Part model, mm, in its own coordinate system. A direction names the side the tool comes from. Round coordinates to 2 decimals unless told otherwise and drop trailing zeros. Loops run counter-clockwise (first coordinate to the right, second up) from the corner with the lowest first, then second, coordinate; pieces in that order, holes last. Notation, with made-up numbers: M -32.5,68.25 L -18.5,68.25 A17 cw -18.5,77.25 Z; hole C 86,41.25 d6. An arc over 180 degrees is marked long. Put each result on its own line as item: value. Start each with the question number.
1) Slice it at C-C on y = 351. Give the cut face in (x, z), then the cut area to 3 significant figures.
2) Drop flat-ended pins along their axis: pin 1 Ø1.2 at (y, z) = (12.5, -0.5) entering from -X; pin 2 Ø3.5 at (x, y) = (29.5, 930) entering from +Z; pin 3 Ø12 at (x, z) = (7, -27) entering from -Y. Give the stop position or say it passes through.
3) Which spindle directions (+Z, -Z, +X, -X, +Y, -Y) get a long thin tool onto all of the face, cutting with end or side? Do faces 1 (the flat face through (1, 20, -20)), 2 (the flat face through (38.5, 602, -20)), 3 (the flat face through (1, 1200, -20)), 4 (the flat face through (20, 601, 0)), 5 (the flat face through (0, 602, -20)). Say none if no direction does.
4) Pull direction X, two halves, no side cores. Call faces 6 (the flat face through (20, 601, -40)), 7 (the flat face through (40, 602, -20)), 8 (the flat face through (20, 601, -1.5)): +X half, -X half, draft (parallel to the pull), parting line (faces both ways), or undercut.
5) Slice it at B-B on z = -28.5. Give the cut face in (x, y), then the cut area to 3 significant figures.
6) Slice it at A-A on x = 13.5. Give the cut face in (y, z), then the cut area to 3 significant figures.
7) Probe line 1 along Z through (x, y) = (7, 613.5); line 2 along X through (y, z) = (69, -11); line 3 along X through (y, z) = (730, -1.1). List the from-to ranges inside material, lowest first.
```python
from build123d import *

# Parameters (mm, degrees)
SKETCH1_W           = 37
SKETCH1_H           = 37
BOSS_EXTRUDE1_DEPTH = 1220
SKETCH2_W           = 20
SKETCH2_H           = 20
SKETCH2_W_2         = 5
CUT_EXTRUDE1_DEPTH  = 50
SKETCH3_R           = 3
CUT_EXTRUDE2_DEPTH  = 10


with BuildPart() as part:
    # Sketch1 → Boss-Extrude1 (new body)
    with BuildSketch(Plane(origin=(0, 0, 0), x_dir=(1, 0, 0), z_dir=(0, 1, 0))):
        with BuildLine():
            Line((0.5, 0), (39.5, 0))
            ThreePointArc((39.5, 0), (39.853553391, 0.146446609), (40, 0.5))
            Line((40, 0.5), (40, 39.5))
            ThreePointArc((40, 39.5), (39.853553391, 39.853553391), (39.5, 40))
            Line((39.5, 40), (0.5, 40))
            ThreePointArc((0.5, 40), (0.146446609, 39.853553391), (0, 39.5))
            Line((0, 39.5), (0, 0.5))
            ThreePointArc((0, 0.5), (0.146446609, 0.146446609), (0.5, 0))
        make_face()
        with Locations((20, 20)):
            Rectangle(SKETCH1_W, SKETCH1_H, mode=Mode.SUBTRACT)
    extrude(amount=BOSS_EXTRUDE1_DEPTH)

    # Sketch2 → Cut-Extrude1 (cut)
    with BuildSketch(Plane.XY):
        with Locations((10, 1210)):
            Rectangle(SKETCH2_W, SKETCH2_H)
        with Locations((37.5, 1210)):
            Rectangle(SKETCH2_W_2, SKETCH2_H)
        with Locations((10, 10)):
            Rectangle(SKETCH2_W, SKETCH2_H)
        with Locations((37.5, 10)):
            Rectangle(SKETCH2_W_2, SKETCH2_H)
    extrude(amount=-CUT_EXTRUDE1_DEPTH, mode=Mode.SUBTRACT)

    # Sketch3 → Cut-Extrude2 (cut)
    with BuildSketch(Plane.XY):
        with Locations((29.5, 90)):
            Circle(SKETCH3_R)
        with Locations((29.5, 290)):
            Circle(SKETCH3_R)
        with Locations((29.5, 490)):
            Circle(SKETCH3_R)
        with Locations(Location((29.5, 730, 0), (0, 0, 180))):
            Circle(SKETCH3_R)
        with Locations(Location((29.5, 930, 0), (0, 0, 180))):
            Circle(SKETCH3_R)
        with Locations(Location((29.5, 1130, 0), (0, 0, 180))):
            Circle(SKETCH3_R)
    extrude(amount=-CUT_EXTRUDE2_DEPTH, mode=Mode.SUBTRACT)


solid = part.part
```
Recorded:
1. outline: M 0,-39.5 A0.5 ccw 0.5,-40 L 39.5,-40 A0.5 ccw 40,-39.5 L 40,-0.5 A0.5 ccw 39.5,0 L 0.5,0 A0.5 ccw 0,-0.5 Z; hole M 1.5,-38.5 L 38.5,-38.5 L 38.5,-1.5 L 1.5,-1.5 Z
1. area: 231 mm2
2. pin 1: stops at x = 20
2. pin 2: stops at z = -38.5
2. pin 3: stops at y = 20
3. face 1: +Z, -Z, -X, -Y
3. face 2: +Y, -Y
3. face 3: +Z, -Z, -X, +Y
3. face 4: +Z, +X, -X, +Y, -Y
3. face 5: +Z, -Z, -X, +Y, -Y
4. face 6: draft
4. face 7: +X half
4. face 8: undercut
5. outline: M 0,20 L 1.5,20 L 1.5,1200 L 0,1200 Z; M 38.5,20 L 40,20 L 40,1200 L 38.5,1200 Z
5. area: 3,540 mm2
6. outline: M 20,-40 L 1200,-40 L 1200,-38.5 L 20,-38.5 Z; M 20,-1.5 L 1200,-1.5 L 1200,0 L 20,0 Z
6. area: 3,540 mm2
7. line 1: z = -40 to -38.5, -1.5 to 0
7. line 2: x = 0 to 1.5, 38.5 to 40
7. line 3: x = 0 to 26.5, 32.5 to 40
